For this review, take the finished solid that the model builds, in its own axes (mm). Round coordinates to 2 decimals unless told otherwise and drop trailing zeros. Write each loop counter-clockwise with the first axis right and the second up, starting at its lowest first coordinate (ties: lowest second). Pieces come first, ordered by that corner, then holes. Notation, with made-up numbers: (74, 51.5) -> (100, 51.5) arc R8 cw to (100, 58.5) -> close; hole circle Ø4 at (48.25, -5.75). An arc over 180 degrees is marked (long way). Write item = value, one per line. Start each with the question number.
```python
from build123d import *

# Parameters (mm, degrees)
BOSS_EXTRUDE1_DEPTH = 3.175
SKETCH2_R           = 3.3782
CUT_EXTRUDE1_DEPTH  = 139.332385308


with BuildPart() as part:
    # Sketch1 → Boss-Extrude1 (new body)
    with BuildSketch(Plane.XY):
        Polygon((0, 0), (0, 97.79), (25.4, 97.79), (25.4, 79.829487758), (25.4, 25.4), (79.829487758, 25.4), (97.79, 25.4), (97.79, 0), align=None)
    extrude(amount=BOSS_EXTRUDE1_DEPTH)

    # Sketch2 → Cut-Extrude1 (cut, through all)
    with BuildSketch(Plane.XY.offset(3.175)):
        with Locations((53.34, 12.7)):
            Circle(SKETCH2_R)
        with Locations((72.39, 12.7)):
            Circle(SKETCH2_R)
        with Locations((12.7, 53.34)):
            Circle(SKETCH2_R)
        with Locations((12.7, 72.39)):
            Circle(SKETCH2_R)
        with Locations((12.7, 91.44)):
            Circle(SKETCH2_R)
        with Locations((91.44, 12.7)):
            Circle(SKETCH2_R)
    extrude(amount=-CUT_EXTRUDE1_DEPTH, mode=Mode.SUBTRACT)


solid = part.part
```
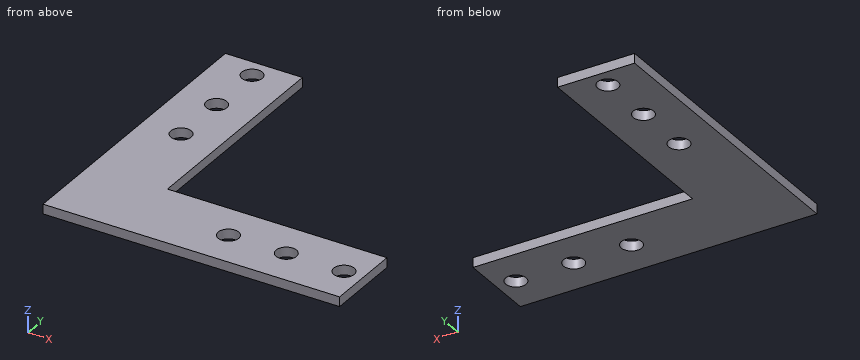
1. Wall thickness on L1, parallel to Y at x = 12.7, z = 2.25; L2, parallel to X at y = 72.5, z = 0.6: over which ranges is each line inside the solid? List them lowest first. Write a range as from..to.
2. Clearance check with flat-ended pins moving along their axes: pin 1 Ø6 at (x, y) = (12.7, 53.34) entering from -Z; pin 2 Ø1 at (x, z) = (57, 1) entering from +Y; pin 3 Ø9 at (x, y) = (91.44, 12.7) entering from +Z (3 decimals). State where each tip first meets the part, or that it passes through.
3. Consider section D-D, the plane x = 12.7. Give the boundary of the cut face in (y, z) (3 decimals).
4. Consider section A-A, the plane y = 91.44. Give the boundary of the cut face in (x, z) (3 decimals), then the cut area to 3 significant figures.
5. Consider section B-B, the plane z = 2.15. Give the boundary of the cut face in (x, y).
Outcome:
q1.L1 = 0..49.96, 56.72..69.01, 75.77..88.06, 94.82..97.79
q1.L2 = 0..9.32, 16.08..25.4
q2.pin_1 = through
q2.pin_2 = 25.4
q2.pin_3 = 3.175
q3.outline = (0, 0) -> (49.962, 0) -> (49.962, 3.175) -> (0, 3.175) -> close; (56.718, 0) -> (69.012, 0) -> (69.012, 3.175) -> (56.718, 3.175) -> close; (75.768, 0) -> (88.062, 0) -> (88.062, 3.175) -> (75.768, 3.175) -> close; (94.818, 0) -> (97.79, 0) -> (97.79, 3.175) -> (94.818, 3.175) -> close
q4.outline = (0, 0) -> (9.322, 0) -> (9.322, 3.175) -> (0, 3.175) -> close; (16.078, 0) -> (25.4, 0) -> (25.4, 3.175) -> (16.078, 3.175) -> close
q4.area = 59.2 mm2
q5.outline = (0, 0) -> (97.79, 0) -> (97.79, 25.4) -> (25.4, 25.4) -> (25.4, 97.79) -> (0, 97.79) -> close; hole circle Ø6.76 at (12.7, 53.34); hole circle Ø6.76 at (12.7, 72.39); hole circle Ø6.76 at (12.7, 91.44); hole circle Ø6.76 at (53.34, 12.7); hole circle Ø6.76 at (72.39, 12.7); hole circle Ø6.76 at (91.44, 12.7)
